Read the model definition and answer for the solid it produces. Units are mm, in the model's axes. A direction names the side the tool comes from. Coordinates: 2 decimals unless noted, no trailing zeros. Loops run counter-clockwise (first coordinate to the right, second up) from the corner with the lowest first, then second, coordinate; pieces in that order, holes last. Notation, with made-up numbers: (-21.5, 17.5) -> (9.5, 17.5) arc R28 cw to (9.5, 47.5) -> close; hole circle Ø1 at (38, 27). An arc over 180 degrees is marked (long way). Answer as a JSON object with one key per item and string values. Group by question number.
1) Section A-A, the plane y = 9.25 is taken. Count the separate pieces of the cut face and the enclosed holes in it, plus the area to 3 significant figures.
2) Section B-B, the plane z = -12 is taken. Give the vertices of the cut face in (x, y) (1 decimal), plus the area to 3 significant figures.
3) Which of the six approach directions +Z, -Z, +X, -X, +Y, -Y give full straight-line access (tool end or side, diameter ignored) to faces 1 (the face through (6.93, -5.31, 10.92)), 2 (the face through (10.6, 3.34, -5.23))?
4) Flat-ended cylindrical pins translate along their axes: P1, Ø6, axis at x = -3, z = 4, coming from the +Y side; P2, Ø3, axis at y = -8.5, z = -15, coming from the +X side; P3, Ø12, axis at x = 8, z = -0.5, coming from the -Y side. Find the tip coordinate at first contact, or state that the pin passes through.
5) Consider probe 1 along X at (y, z) = (-0.25, 13.5); probe 2 along Y at (x, z) = (0, -14.5). Determine where each line is inside the solid, lowest interval first. Write a range as [from, to].
6) Section D-D, the plane z = 12 is taken. Give the vertices of the cut face in (x, y) (1 decimal), plus the area to 3 significant figures.
7) Determine the mould class of faces 3 (the face through (6.93, -5.31, -14.99)), 4 (the face through (-3.78, -2.9, -1.25)), 5 (the face through (7, -6, 0.381)) for opening direction Y: released by +Y, released by -Y, zero draft, split by the parting line, or undercut.
from build123d import *

# Parameters (mm, degrees)
SKETCH1_R          = 11.1125
SKETCH1_R_2        = 3.2004
EXTRUDE1_DEPTH     = 25.4
SKETCH5_R          = 11.1125
SKETCH5_R_2        = 3.2004
CUT_EXTRUDE1_DEPTH = 3.175
SKETCH6_R          = 4.7625
CUT_EXTRUDE2_DEPTH = 48.625
CUT_EXTRUDE3_START = -1.5875
SKETCH7_R          = 11.1125
SKETCH7_R_2        = 8.73125
CUT_EXTRUDE3_DEPTH = 4.7625
LPATTERN1_COUNT    = 6
LPATTERN1_PITCH    = 6.477


with BuildPart() as part:
    # Sketch1 → Extrude1 (new body, symmetric)
    with BuildSketch(Plane.XY):
        Circle(SKETCH1_R)
        Circle(SKETCH1_R_2, mode=Mode.SUBTRACT)
    extrude(amount=EXTRUDE1_DEPTH, both=True)

    # Sketch5 → Cut-Extrude1 (cut)
    with BuildSketch(Plane.XY.offset(25.4)):
        Circle(SKETCH5_R)
        Circle(SKETCH5_R_2, mode=Mode.SUBTRACT)
    extrude(amount=-CUT_EXTRUDE1_DEPTH, mode=Mode.SUBTRACT)

    # Sketch6 → Cut-Extrude2 (cut, through all)
    with BuildSketch(Plane.XY.offset(22.225)):
        Circle(SKETCH6_R)
    extrude(amount=-CUT_EXTRUDE2_DEPTH, mode=Mode.SUBTRACT)

    # Sketch7 → Cut-Extrude3 (cut)
    with BuildSketch(Plane(origin=(0, 0, -25.4), x_dir=(-1, 0, 0), z_dir=(0, 0, -1)).offset(CUT_EXTRUDE3_START)):
        Circle(SKETCH7_R)
        Circle(SKETCH7_R_2, mode=Mode.SUBTRACT)
    cut_extrude3 = extrude(amount=-CUT_EXTRUDE3_DEPTH, mode=Mode.SUBTRACT)

    # LPattern1: Cut-Extrude3 ×6
    with Locations(*[(0, 0, i * LPATTERN1_PITCH) for i in range(1, LPATTERN1_COUNT)]):
        add(cut_extrude3, mode=Mode.SUBTRACT)


solid = part.part
Determined:
{
 "1": {"separate pieces": "7", "enclosed holes": "0", "area": "235 mm²"},
 "2": {"outline": "circle Ø22.2 at (0, 0); hole circle Ø9.5 at (0, 0)", "area": "317 mm²"},
 "3": {"face 1": "none", "face 2": "+Z, -Z"},
 "4": {"P1": "y = 11.09", "P2": "x = 5.22", "P3": "y = -10.92"},
 "5": {"probe 1": "[-11.11, -4.76], [4.76, 11.11]", "probe 2": "[-8.73, -4.76], [4.76, 8.73]"},
 "6": {"outline": "circle Ø17.5 at (0, 0); hole circle Ø9.5 at (0, 0)", "area": "168 mm²"},
 "7": {"face 3": "split by the parting line", "face 4": "undercut", "face 5": "zero draft"}
}
